```python
from build123d import *

# Parameters (mm, degrees)
BOSS_EXTRUDE1_DEPTH = 1
SKETCH1_4_R         = 5.5
SKETCH1_4_R_2       = 4.5
BOSS_EXTRUDE2_DEPTH = 2


with BuildPart() as part:
    # Sketch1 → Boss-Extrude1 (new body)
    with BuildSketch(Plane.XY):
        with BuildLine():
            Line((-8.649421946, -5.5), (8.649421946, -5.5))
            ThreePointArc((8.649421946, -5.5), (0, 10.25), (-8.649421946, -5.5))
        make_face()
    extrude(amount=BOSS_EXTRUDE1_DEPTH)

    # Sketch1<4> → Boss-Extrude2 (add)
    with BuildSketch(Plane.XY):
        Circle(SKETCH1_4_R)
        Circle(SKETCH1_4_R_2, mode=Mode.SUBTRACT)
    extrude(amount=-BOSS_EXTRUDE2_DEPTH)


solid = part.part
```
Read the model definition and answer for the solid it produces. Units are mm, in the model's axes. A direction names the side the tool comes from. Coordinates: 2 decimals unless noted, no trailing zeros. Write each loop counter-clockwise with the first axis right and the second up, starting at its lowest first coordinate (ties: lowest second). Pieces come first, ordered by that corner, then holes. Notation, with made-up numbers: (77.5, 74.25) -> (119.5, 74.25) arc R26 cw to (119.5, 108.25) -> close; hole circle Ø5 at (88, 57). An arc over 180 degrees is marked (long way). Return JSON: item names as keys, results as strings.
1. Find the intervals of material crossed by line 1 along Y through (x, z) = (0, -1.4); line 2 along X through (y, z) = (3.25, -0.5); line 3 along X through (y, z) = (-0.25, 0.8), in increasing order. Write a range as from..to.
Found:
{"line 1": "-5.5..-4.5, 4.5..5.5", "line 2": "-4.44..-3.11, 3.11..4.44", "line 3": "-10.25..10.25"}
2. This flat-tipped pin is pushed along its axis until it touches: P1, Ø8, axis at x = 0, y = 0, coming from the -Z side. Where does it stop, or does it pass through?
Found:
{"P1": "z = 0"}
3. A cutting plane is placed at D-D (x = -8). Determine the outline of the cut face in (y, z).
Found:
{"outline": "(-5.5, 0) -> (6.41, 0) -> (6.41, 1) -> (-5.5, 1) -> close"}
4. A cutting plane is placed at A-A (y = 0). Determine the outline of the cut face in (x, z).
Found:
{"outline": "(-10.25, 0) -> (-5.5, 0) -> (-5.5, -2) -> (-4.5, -2) -> (-4.5, 0) -> (4.5, 0) -> (4.5, -2) -> (5.5, -2) -> (5.5, 0) -> (10.25, 0) -> (10.25, 1) -> (-10.25, 1) -> close"}
5. A cutting plane is placed at C-C (z = -0.45). Determine the outline of the cut face in (x, y).
Found:
{"outline": "circle Ø11 at (0, 0); hole circle Ø9 at (0, 0)"}
6. A tool of negligible diameter and unlimited length cuts with its end or side. For faces 1 (the face through (0.307, 10.245, 0.493)), 2 (the face through (-1.19, -5.37, -0.99)), from which of +Z, -Z, +X, -X, +Y, -Y can it reach the whole face along a straight path? Write none if from no direction.
Found:
{"face 1": "+Z, -Z", "face 2": "-Z"}
